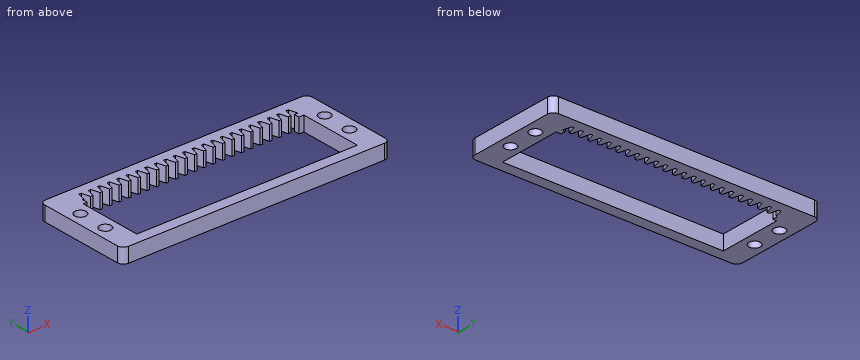
from build123d import *

# Parameters (mm, degrees)
BOSS_EXTRUDE1_DEPTH = 5
SKETCH2_W           = 75
SKETCH2_H           = 21.5
CUT_EXTRUDE1_DEPTH  = 6
SKETCH3_W           = 71.97
SKETCH3_H           = 1.85
CUT_EXTRUDE2_DEPTH  = 6
CUT_EXTRUDE4_DEPTH  = 6
LPATTERN1_COUNT     = 23
LPATTERN1_PITCH     = 3.2
SKETCH5_R           = 1.95
CUT_EXTRUDE5_DEPTH  = 10


with BuildPart() as part:
    # Sketch1 → Boss-Extrude1 (new body)
    with BuildSketch(Plane.XY):
        with BuildLine():
            Line((2, 0), (89, 0))
            ThreePointArc((89, 0), (90.414213562, -0.585786438), (91, -2))
            Line((91, -2), (91, -31.22))
            ThreePointArc((91, -31.22), (90.414213562, -32.634213562), (89, -33.22))
            Line((89, -33.22), (2, -33.22))
            ThreePointArc((2, -33.22), (0.585786438, -32.634213562), (0, -31.22))
            Line((0, -31.22), (0, -2))
            ThreePointArc((0, -2), (0.585786438, -0.585786438), (2, 0))
        make_face()
    extrude(amount=BOSS_EXTRUDE1_DEPTH)

    # Sketch2 → Cut-Extrude1 (cut, through all)
    with BuildSketch(Plane.XY.offset(5)):
        with Locations((45.5, -18.75)):
            Rectangle(SKETCH2_W, SKETCH2_H)
    extrude(amount=-CUT_EXTRUDE1_DEPTH, mode=Mode.SUBTRACT)

    # Sketch3 → Cut-Extrude2 (cut, through all)
    with BuildSketch(Plane.XY.offset(5)):
        with Locations((45.335, -7.075)):
            Rectangle(SKETCH3_W, SKETCH3_H)
    extrude(amount=-CUT_EXTRUDE2_DEPTH, mode=Mode.SUBTRACT)

    # Sketch4 → Cut-Extrude4 (cut, through all)
    with BuildSketch(Plane.XY.offset(5)):
        Polygon((81.735, -3.249176841), (82.5, -6.15), (80.14, -6.15), (80.905, -3.249176841), align=None)
    cut_extrude4 = extrude(amount=-CUT_EXTRUDE4_DEPTH, mode=Mode.SUBTRACT)

    # LPattern1: Cut-Extrude4 ×23
    with Locations(*[(-i * LPATTERN1_PITCH, 0, 0) for i in range(1, LPATTERN1_COUNT)]):
        add(cut_extrude4, mode=Mode.SUBTRACT)

    # Sketch5 → Cut-Extrude5 (cut)
    with BuildSketch(Plane.XY.offset(5)):
        with Locations((4, -11.61)):
            Circle(SKETCH5_R)
        with Locations((4, -21.61)):
            Circle(SKETCH5_R)
        with Locations((87, -11.61)):
            Circle(SKETCH5_R)
        with Locations((87, -21.61)):
            Circle(SKETCH5_R)
    extrude(amount=-CUT_EXTRUDE5_DEPTH, mode=Mode.SUBTRACT)


solid = part.part
Geometry: final body of the model. Coordinates: model frame, mm. Give positions to 0.01 mm unless a question says otherwise; leave off trailing zeros. Order: outer loops, then holes, each group sorted by start corner. A loop starts at its lowest first (then second) coordinate and runs counter-clockwise, first axis right, second up. Notation, with made-up numbers: (-1, 2.5) - (23, 2.5) arc R5 cw to (23, 8.5) - close; hole circle Ø8 at (2, -36). An arc over 180 degrees is marked (long way). Use CSV: the item, a comma, the result in double quotes.
1. Section query D-D (z = 1.8). Give the number of separate pieces and of enclosed holes in the cut face, plus the area to 3 significant figures.
Answers below:
separate pieces,"1"
enclosed holes,"5"
area,"1,120 mm2"
2. Section query B-B (y = -17.5). Output: boundary loops of the cut face in (x, z), plus the area to 3 significant figures.
Answers below:
outline,"(0, 0) - (8, 0) - (8, 5) - (0, 5) - close; (83, 0) - (91, 0) - (91, 5) - (83, 5) - close"
area,"80.0 mm2"
3. Section query C-C (x = 4). Output: boundary loops of the cut face in (y, z).
Answers below:
outline,"(-33.22, 0) - (-23.56, 0) - (-23.56, 5) - (-33.22, 5) - close; (-19.66, 0) - (-13.56, 0) - (-13.56, 5) - (-19.66, 5) - close; (-9.66, 0) - (0, 0) - (0, 5) - (-9.66, 5) - close"
4. Section query A-A (y = -11.61). Output: boundary loops of the cut face in (x, z).
Answers below:
outline,"(0, 0) - (2.05, 0) - (2.05, 5) - (0, 5) - close; (5.95, 0) - (8, 0) - (8, 5) - (5.95, 5) - close; (83, 0) - (85.05, 0) - (85.05, 5) - (83, 5) - close; (88.95, 0) - (91, 0) - (91, 5) - (88.95, 5) - close"
5. Material intervals for line 1 along Y through (x, z) = (87, 3.25); line 2 along X through (y, z) = (-23, 3.5); line 3 along X through (y, z) = (-26.5, 0.9), sorted ascending. Write a range as from..to.
Answers below:
line 1,"-33.22..-23.56, -19.66..-13.56, -9.66..0"
line 2,"0..2.63, 5.37..8, 83..85.63, 88.37..91"
line 3,"0..8, 83..91"
6. Contact query for a flat-ended pin moving along its axis: pin 1 (3.5 mm diameter, centred on x = 87, y = -11.61, fed in from +Z). Output: stop coordinate, or through.
Answers below:
pin 1,"through"
